from build123d import *

# Parameters (mm, degrees)
BOSS_EXTRUDE1_DEPTH            = 30.5
CUT_EXTRUDE1_START             = 30.5
CUT_EXTRUDE1_DEPTH             = 5
CBORE_FOR_M4_SHCS1_D           = 4.5
CBORE_FOR_M4_SHCS1_CBORE_D     = 9.7
CBORE_FOR_M4_SHCS1_CBORE_DEPTH = 55.5
F_1_4_20_TAPPED_HOLE1_D        = 5.1054
F_1_4_20_TAPPED_HOLE1_DEPTH    = 12
FILLET1_R                      = 10
SKETCH8_W                      = 15.1
SKETCH8_H                      = 20.9
BOSS_EXTRUDE2_DEPTH            = 5


with BuildPart() as part:
    # Sketch1 → Boss-Extrude1 (new body, symmetric)
    with BuildSketch(Plane.XY):
        with BuildLine():
            Line((-49, 131), (49, 131))
            ThreePointArc((49, 131), (77.284271247, 119.284271247), (89, 91))
            Line((89, 91), (89, -91))
            ThreePointArc((89, -91), (77.284271247, -119.284271247), (49, -131))
            Line((49, -131), (-49, -131))
            ThreePointArc((-49, -131), (-77.284271247, -119.284271247), (-89, -91))
            Line((-89, -91), (-89, 91))
            ThreePointArc((-89, 91), (-77.284271247, 119.284271247), (-49, 131))
        make_face()
    extrude(amount=BOSS_EXTRUDE1_DEPTH, both=True)

    # Sketch1<4> → Cut-Extrude1 (cut)
    with BuildSketch(Plane.XY.offset(CUT_EXTRUDE1_START)):
        with BuildLine():
            Line((-29.05, 11.25), (29.05, 11.25))
            ThreePointArc((29.05, 11.25), (29.757106781, 10.957106781), (30.05, 10.25))
            Line((30.05, 10.25), (30.05, -33.25))
            ThreePointArc((30.05, -33.25), (29.757106781, -33.957106781), (29.05, -34.25))
            Line((29.05, -34.25), (-29.05, -34.25))
            ThreePointArc((-29.05, -34.25), (-29.757106781, -33.957106781), (-30.05, -33.25))
            Line((-30.05, -33.25), (-30.05, 10.25))
            ThreePointArc((-30.05, 10.25), (-29.757106781, 10.957106781), (-29.05, 11.25))
        make_face()
    extrude(amount=-CUT_EXTRUDE1_DEPTH, mode=Mode.SUBTRACT)

    # CBORE for M4 SHCS1 (through all)
    with Locations(Plane.XY.offset(30.5)):
        with Locations((-44.6, -11.5), (44.6, -11.5)):
            CounterBoreHole(CBORE_FOR_M4_SHCS1_D / 2, CBORE_FOR_M4_SHCS1_CBORE_D / 2, CBORE_FOR_M4_SHCS1_CBORE_DEPTH)

    # 1/4-20 Tapped Hole1
    with Locations(Plane(origin=(0, 0, -30.5), x_dir=(-1, 0, 0), z_dir=(0, 0, -1))):
        with Locations((0, 12)):
            Hole(F_1_4_20_TAPPED_HOLE1_D / 2, depth=F_1_4_20_TAPPED_HOLE1_DEPTH)

    # Sketch4 → Revolve1 (revolve)
    with BuildSketch(Plane(origin=(0, 0, 0), x_dir=(0, 0, -1), z_dir=(1, 0, 0))):
        with BuildLine():
            Line((-36.4, -109), (-9.991525424, -109))
            ThreePointArc((-9.991525424, -109), (-23.195762712, -95.795762712), (-36.4, -109))
        make_face()
    revolve(axis=Axis((0, -109, 157.281610428), (0, 0, -1)))

    # Fillet1
    fillet1_edges = [part.edges().sort_by_distance(p)[0] for p in [
        (77.284271247, 119.284271247, -30.5),
        (0, 131, 30.5),
        (89, 0, -30.5),
        (77.284271247, -119.284271247, -30.5),
        (0, -131, -30.5),
        (-77.284271247, -119.284271247, -30.5),
        (-89, 0, -30.5),
        (-77.284271247, 119.284271247, -30.5),
        (0, 131, -30.5),
        (-77.284271247, 119.284271247, 30.5),
        (-89, 0, 30.5),
        (-77.284271247, -119.284271247, 30.5),
        (0, -131, 30.5),
        (77.284271247, -119.284271247, 30.5),
        (89, 0, 30.5),
        (77.284271247, 119.284271247, 30.5),
    ]]
    fillet(fillet1_edges, radius=FILLET1_R)

    # Sketch8 → Boss-Extrude2 (add)
    with BuildSketch(Plane.ZY.offset(89)):
        with Locations((0, 70.55)):
            Rectangle(SKETCH8_W, SKETCH8_H)
    extrude(amount=BOSS_EXTRUDE2_DEPTH)


solid = part.part
Could you check a few things on this model? Use its own coordinates, in mm. A direction names the side the tool comes from. Give positions to 0.01 mm unless a question says otherwise; leave off trailing zeros. Order: outer loops, then holes, each group sorted by start corner. A loop starts at its lowest first (then second) coordinate and runs counter-clockwise, first axis right, second up.
1. We'd pull the mould along X, two halves only. Please class faces 5 (the flat face through (-30.05, -12, 28)), 6 (the flat face through (0, 12, -18.5)), 7 (the flat face through (-94, 71, 0)), 8 (the cylindrical face through (76.972, 119.594, 0.287)): pulls with the +X half, pulls with the -X half, needs draft (parallel to the pull), parting line crosses it, or undercut.
2. I need wall thicknesses on L1, parallel to Y at x = 0, z = -21.25; L2, parallel to Y at x = 44, z = -13; L3, parallel to X at y = -5, z = 10. Which ranges of each line are inside material? Lowest first, please.
3. Suppose I cut it at A-A (z = -1). List the corners of the cut face in (x, y) for me.
4. Will these pins go through, and if not, where does the flat tip stop? P1, Ø4.5, axis at x = 0, y = 12, coming from the +Z side; P2, Ø2.5, axis at x = -44.6, y = -11.5, coming from the +Z side; P3, Ø5.5, axis at x = 9, z = 28, coming from the -Y side; P4, Ø6, axis at y = -16.5, z = 0.5, coming from the -X side.
5. For faces 1 (the flat face through (0, 11.25, 28)), 2 (the flat face through (-91, 70, 7.55)), 3 (the cylindrical face through (-0.553, 9.508, -24.416)), 4 (the cylindrical face through (-77.594, 118.972, 0.287)), which set-ups out of +Z, -Z, +X, -X, +Y, -Y let a thin tool reach every point of the face, with its end or its side?
6. Suppose I cut it at B-B (z = 13). List the corners of the cut face in (x, y) for me, plus the area to 3 significant figures.
Solved:
1. face 5: undercut
1. face 6: undercut
1. face 7: pulls with the -X half
1. face 8: pulls with the +X half
2. L1: y = -130.97 to 9.45, 14.55 to 130.97
2. L2: y = -131 to -16.31, -6.69 to 131
2. L3: x = -89 to 89
3. outline: (-94, 60.1) - (-89, 60.1) - (-89, -91) arc R40 ccw to (-49, -131) - (49, -131) arc R40 ccw to (89, -91) - (89, 91) arc R40 ccw to (49, 131) - (-49, 131) arc R40 ccw to (-89, 91) - (-89, 81) - (-94, 81) - close; hole circle Ø9.7 at (-44.6, -11.5); hole circle Ø9.7 at (44.6, -11.5)
4. P1: stops at z = 30.5
4. P2: passes through
4. P3: stops at y = -129.8
4. P4: stops at x = -89
5. face 1: +Z
5. face 2: +Z, -X, +Y, -Y
5. face 3: -Z
5. face 4: +Z, -Z, -X, +Y
6. outline: (-89, -91) arc R40 ccw to (-49, -131) - (49, -131) arc R40 ccw to (89, -91) - (89, 91) arc R40 ccw to (49, 131) - (-49, 131) arc R40 ccw to (-89, 91) - close; hole circle Ø9.7 at (-44.6, -11.5); hole circle Ø9.7 at (44.6, -11.5)
6. area: 45,100 mm2
